```python
from build123d import *

# Parameters (mm, degrees)
BOSS_EXTRUDE1_DEPTH = 116
LPATTERN1_COUNT     = 5
LPATTERN1_PITCH     = 50


with BuildPart() as part:
    # Sketch1 → Boss-Extrude1 (new, symmetric)
    with BuildSketch(Plane(origin=(0, 0, 0), x_dir=(0, 0, -1), z_dir=(1, 0, 0))):
        Polygon((0, 0), (9.326153163099908, 19.999999999999996), (4.326153163099911, 19.999999999999996), (-5.000000000000001, -8.7e-16), align=None)
    extrude(amount=BOSS_EXTRUDE1_DEPTH, both=True)

    # Sketch3 → Cut-Revolve1 (revolve, cut)
    with BuildSketch(Plane.ZY.offset(103.00000000000001)):
        Polygon((-1.5444404272329906, 8.999999999999998), (2.854482547232013, 4.601077025535014), (0.8032310766050411, 8.999999999999998), align=None)
    cut_revolve1 = revolve(axis=Axis((-103.00000000000001, 9.000000000000002, 9.024012903581264), (0, -1.5e-16, -1)), mode=Mode.SUBTRACT)

    # LPattern1: Cut-Revolve1 ×5
    with Locations(*[(i * LPATTERN1_PITCH, 0, 0) for i in range(1, LPATTERN1_COUNT)]):
        add(cut_revolve1, mode=Mode.SUBTRACT)


solid = part.part
```
Model file for the job. Use its own axes, mm. Give positions to 0.01 mm unless a question says otherwise; leave off trailing zeros. Write each loop counter-clockwise with the first axis right and the second up, starting at its lowest first coordinate (ties: lowest second). Pieces come first, ordered by that corner, then holes. Notation, with made-up numbers: (12.25, -9) - (55.25, -9) arc R24 cw to (55.25, 25) - close; hole circle Ø9 at (46, 83). An arc over 180 degrees is marked (long way). One line per question, with ' | ' between items. Start each with the question number.
(1) Slice it at A-A on x = 67. Write the cut outline in (y, z), plus the area to 3 significant figures.
(2) Wall check: line 1 along Z through (x, y) = (105.5, 11.5); line 2 along Z through (x, y) = (-63, 13); line 3 along Y through (x, z) = (-44, -2). Give the ranges that are in metal, low to high. Write a range as from..to.
(3) Two-plate mould, pull along Y, no slides. Class faces 1 (the face through (96.624, 7.805, -0.292)), 2 (the face through (1.62, 10.14, 0.27)), 3 (the face through (1.62, 9.86, -4.6)): +Y half, -Y half, draft (parallel to the pull), parting line (faces both ways), or undercut.
(4) Pin check, flat tips, straight feed: P1, Ø3, axis at x = 11, z = -0.5, coming from the +Y side; P2, Ø6, axis at x = 34, y = 16, coming from the -Z side; P3, Ø2, axis at x = -50.5, z = -6.5, coming from the -Y side. Stop position of each tip, or through.
Results below:
1) outline: (0, 0) - (20, -9.33) - (20, -4.33) - (0, 5) - close | area: 100 mm^2
2) line 1: -5.36..-0.36 | line 2: -6.06..-1.06 | line 3: 4.29..15.01
3) face 1: undercut | face 2: +Y half | face 3: -Y half
4) P1: y = 15.01 | P2: z = -8.86 | P3: y = 11.79
